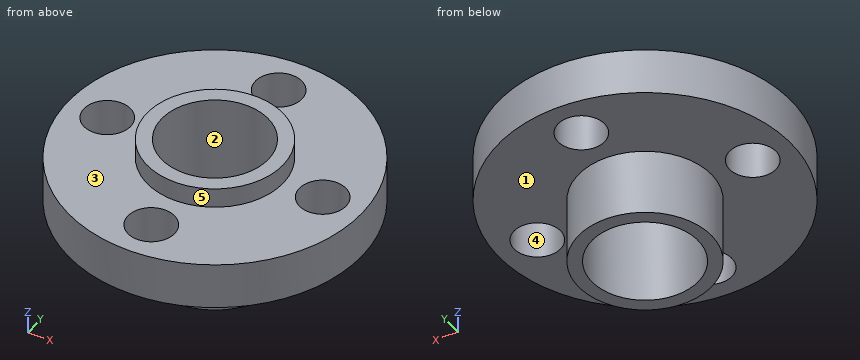
```python
from build123d import *

# Parameters (mm, degrees)
SKETCH_1_R          = 11
SKETCH_1_R_2        = 1.75
EXTRUDE_2_DEPTH     = 3.5
SKETCH_2_R          = 5.1
EXTRUDE_4_DEPTH     = 1.5
SKETCH_3_R          = 5
EXTRUDE_5_DEPTH     = 5
SKETCH_4_R          = 4
CUT_EXTRUDE_4_DEPTH = 11


with BuildPart() as part:
    # 草圖1 → 填料-伸長2 (new body)
    with BuildSketch(Plane.XY):
        Circle(SKETCH_1_R)
        with Locations((0, 8)):
            Circle(SKETCH_1_R_2, mode=Mode.SUBTRACT)
        with Locations((8, 0)):
            Circle(SKETCH_1_R_2, mode=Mode.SUBTRACT)
        with Locations((0, -8)):
            Circle(SKETCH_1_R_2, mode=Mode.SUBTRACT)
        with Locations((-8, 0)):
            Circle(SKETCH_1_R_2, mode=Mode.SUBTRACT)
    extrude(amount=EXTRUDE_2_DEPTH)

    # 草圖2 → 填料-伸長4 (add)
    with BuildSketch(Plane.XY.offset(3.5)):
        Circle(SKETCH_2_R)
    extrude(amount=EXTRUDE_4_DEPTH)

    # 草圖3 → 填料-伸長5 (add)
    with BuildSketch(Plane(origin=(0, 0, 0), x_dir=(-1, 0, 0), z_dir=(0, 0, -1))):
        Circle(SKETCH_3_R)
    extrude(amount=EXTRUDE_5_DEPTH)

    # 草圖4 → 除料-伸長4 (cut, through all)
    with BuildSketch(Plane.XY.offset(5)):
        Circle(SKETCH_4_R)
    extrude(amount=-CUT_EXTRUDE_4_DEPTH, mode=Mode.SUBTRACT)


solid = part.part
```
Check sheet for the modelled part. Datum: model origin and axes. Units: mm. Face numbers are marked on the shaded views. A direction names the side the tool comes from. Round coordinates to 2 decimals unless told otherwise and drop trailing zeros. Write each loop counter-clockwise with the first axis right and the second up, starting at its lowest first coordinate (ties: lowest second). Pieces come first, ordered by that corner, then holes. Notation, with made-up numbers: (47, -26) -> (99, -26) arc R17 ccw to (99, -20) -> close; hole circle Ø2 at (11.5, 77.5). An arc over 180 degrees is marked (long way). One line per question, with ' | ' between items. Start each with the question number.
1. Depth check by flat-ended pin: pin 1 (4 mm diameter, centred on x = 0, y = 8, fed in from +Z); pin 2 (4 mm diameter, centred on y = 8.5, z = 1.5, fed in from -X); pin 3 (2 mm diameter, centred on x = -5, z = 3.5, fed in from +Y). Enter the tip coordinate at first touch or a pass-through.
2. Scan lines: line 1 along Y through (x, z) = (0, 2.7); line 2 along X through (y, z) = (-1, -3.75); line 3 along Z through (x, y) = (7, 6). Record each from-to range of solid material in increasing order. Write a range as from..to.
3. Set-up check for the marked faces 1 and 2: record each of +Z, -Z, +X, -X, +Y, -Y from which the full face is reachable in a straight line by a thin tool's end or side.
4. Sectioned sample at C-C, the plane z = 2. Record the cut outline in (x, y).
5. Release check for a two-part mould opening along Y. For the marked faces 3, 4 and 5 record: +Y half, -Y half, draft (parallel to the pull), parting line (faces both ways), or undercut.
6. Sectioned sample at A-A, the plane y = 0. Record the cut outline in (x, z).
7. Sectioned sample at D-D, the plane y = 8. Record the cut outline in (x, z).
Taken from the geometry:
1) pin 1: stops at z = 3.5 | pin 2: stops at x = -8.87 | pin 3: stops at y = 10.25
2) line 1: y = -11..-9.75, -6.25..-4, 4..6.25, 9.75..11 | line 2: x = -4.9..-3.87, 3.87..4.9 | line 3: z = 0..3.5
3) face 1: -Z | face 2: +Z, -Z
4) outline: circle Ø22 at (0, 0); hole circle Ø3.5 at (-8, 0); hole circle Ø8 at (0, 0); hole circle Ø3.5 at (0, -8); hole circle Ø3.5 at (0, 8); hole circle Ø3.5 at (8, 0)
5) face 3: draft | face 4: undercut | face 5: parting line
6) outline: (-11, 0) -> (-9.75, 0) -> (-9.75, 3.5) -> (-11, 3.5) -> close; (-6.25, 0) -> (-5, 0) -> (-5, -5) -> (-4, -5) -> (-4, 5) -> (-5.1, 5) -> (-5.1, 3.5) -> (-6.25, 3.5) -> close; (4, -5) -> (5, -5) -> (5, 0) -> (6.25, 0) -> (6.25, 3.5) -> (5.1, 3.5) -> (5.1, 5) -> (4, 5) -> close; (9.75, 0) -> (11, 0) -> (11, 3.5) -> (9.75, 3.5) -> close
7) outline: (-7.55, 0) -> (-1.75, 0) -> (-1.75, 3.5) -> (-7.55, 3.5) -> close; (1.75, 0) -> (7.55, 0) -> (7.55, 3.5) -> (1.75, 3.5) -> close
